from build123d import *

# Parameters (mm, degrees)
F0_R     = 14.22
F0_W     = 12.87
F0_H     = 5.35
F1_DEPTH = 2


with BuildPart() as f1:
    # F0 (on Front) → F1 (new body)
    with BuildSketch(Plane.XZ):
        Circle(F0_R)
        with Locations((0, -4.26)):
            Rectangle(F0_W, F0_H, mode=Mode.SUBTRACT)
        with Locations((0, 4.26)):
            Rectangle(F0_W, F0_H, mode=Mode.SUBTRACT)
    extrude(amount=F1_DEPTH)


solid = f1.part
Source: CAD feature listing. Evaluate the final solid. Frame: model axes, mm. A direction names the side the tool comes from. Round coordinates to 2 decimals unless told otherwise and drop trailing zeros. Loops run counter-clockwise (first coordinate to the right, second up) from the corner with the lowest first, then second, coordinate; pieces in that order, holes last. Notation, with made-up numbers: (-29, 46) - (6, 46) arc R14 ccw to (6, 73) - close; hole circle Ø2 at (-32.75, 50.25). An arc over 180 degrees is marked (long way). Write item = value, one per line. Start each with the question number.
(1) Section query A-A, the plane x = 0. Output: boundary loops of the cut face in (y, z) (3 decimals), plus the area to 3 significant figures.
(2) Section query C-C, the plane z = -4.5. Output: boundary loops of the cut face in (x, y) (3 decimals).
(3) Pull-direction query (Z, two-part tool) for faces 3 (the face through (0, -1, 1.585)), 4 (the face through (13.563, -0.986, 4.271)), 5 (the face through (0, -2, 0)); classes: +Z half, -Z half, draft (parallel to the pull), parting line (faces both ways), or undercut.
(4) Ray query, line 1 along Z through (x, y) = (-2.5, -0.9) (3 decimals); line 2 along Z through (x, y) = (-3, -1.7) (3 decimals); line 3 along X through (y, z) = (-1.45, 6.25) (3 decimals). Return the intervals inside material, ascending. Write a range as from..to.
(5) Pin query (flat end, axial travel): pin 1 (1 mm diameter, centred on x = 3, y = -0.5, fed in from +Z); pin 2 (0.6 mm diameter, centred on y = -1, z = 5, fed in from -X). Return the tip coordinate at first contact, or that it passes through.
(6) Section query D-D, the plane x = 3.75. Output: boundary loops of the cut face in (y, z) (3 decimals), plus the area to 3 significant figures.
(7) Set-up query: faces 1 (the face through (0, 0, 0)), 2 (the face through (6.435, -1, -4)). Return all of +Z, -Z, +X, -X, +Y, -Y with unobstructed straight access to the full face (end or side cutting, diameter ignored); none if empty.
(8) Section query B-B, the plane y = -1.05. Output: boundary loops of the cut face in (x, z) (3 decimals).
Conclusion:
q1.outline = (-2, -14.22) - (0, -14.22) - (0, -6.935) - (-2, -6.935) - close; (-2, -1.585) - (0, -1.585) - (0, 1.585) - (-2, 1.585) - close; (-2, 6.935) - (0, 6.935) - (0, 14.22) - (-2, 14.22) - close
q1.area = 35.5 mm2
q2.outline = (-13.489, -2) - (-6.435, -2) - (-6.435, 0) - (-13.489, 0) - close; (6.435, -2) - (13.489, -2) - (13.489, 0) - (6.435, 0) - close
q3.face_3 = undercut
q3.face_4 = parting line
q3.face_5 = draft
q4.line_1 = -13.999..-6.935, -1.585..1.585, 6.935..13.999
q4.line_2 = -13.9..-6.935, -1.585..1.585, 6.935..13.9
q4.line_3 = -12.773..-6.435, 6.435..12.773
q5.pin_1 = 14
q5.pin_2 = -13.42
q6.outline = (-2, -13.717) - (0, -13.717) - (0, -6.935) - (-2, -6.935) - close; (-2, -1.585) - (0, -1.585) - (0, 1.585) - (-2, 1.585) - close; (-2, 6.935) - (0, 6.935) - (0, 13.717) - (-2, 13.717) - close
q6.area = 33.5 mm2
q7.face_1 = +Z, -Z, +X, -X, +Y
q7.face_2 = +Y, -Y
q8.outline = circle Ø28.44 at (0, 0); hole (-6.435, -6.935) - (6.435, -6.935) - (6.435, -1.585) - (-6.435, -1.585) - close; hole (-6.435, 1.585) - (6.435, 1.585) - (6.435, 6.935) - (-6.435, 6.935) - close
